```python
from build123d import *

# Parameters (mm, degrees)
SKETCH_1_W               = 15
SKETCH_1_H               = 15
EXTRUDE_1_DEPTH          = 5.5
CUT_EXTRUDE_1_DEPTH      = 11
EXTRUDE_2_DEPTH          = 2
EXTRUDE_2_DEPTH_BACK     = 2
CUT_EXTRUDE_2_DEPTH      = 2
CUT_EXTRUDE_2_DEPTH_BACK = 2
SKETCH_5_W               = 5.4
SKETCH_5_H               = 7.4
EXTRUDE_3_DEPTH          = 1
SKETCH_6_W               = 5.4
SKETCH_6_H               = 5
EXTRUDE_4_DEPTH          = 2
SKETCH_7_R               = 2
EXTRUDE_5_DEPTH          = 10
SKETCH_8_R               = 2.1
EXTRUDE_6_DEPTH          = 1
CHAMFER_1_SIZE           = 0.5
SKETCH_9_W               = 5
SKETCH_9_H               = 1
CUT_EXTRUDE_3_DEPTH      = 6
FILLET_1_R               = 0.1
FILLET_2_R               = 0.2


with BuildPart() as part:
    # 草图1 → 凸台-拉伸1 (new body)
    with BuildSketch(Plane(origin=(0, 0, 0), x_dir=(1, 0, 0), z_dir=(0, 1, 0))):
        Rectangle(SKETCH_1_W, SKETCH_1_H)
    extrude(amount=EXTRUDE_1_DEPTH)

    # 草图2 → 切除-拉伸1 (cut)
    with BuildSketch(Plane.XY.offset(7.5)):
        with BuildLine():
            Line((1.5, 0), (-1.5, 0))
            Line((-1.5, 0), (-1.5, 0.677124344))
            ThreePointArc((-1.5, 0.677124344), (0, 4), (1.5, 0.677124344))
            Line((1.5, 0.677124344), (1.5, 0))
        make_face()
    extrude(amount=-CUT_EXTRUDE_1_DEPTH, mode=Mode.SUBTRACT)

    # 草图3 → 凸台-拉伸2 (add, two sides: drawn at the far end of the back side and taken through both)
    with BuildSketch(Plane.XY.offset(-EXTRUDE_2_DEPTH_BACK)):
        with BuildLine():
            Line((1.5, 5.5), (-1.5, 5.5))
            Line((-1.5, 5.5), (-1.5, 6.177124344))
            ThreePointArc((-1.5, 6.177124344), (-1.780042303, 6.588161527), (-1.95, 7.055590279))
            Line((-1.95, 7.055590279), (-1.95, 8))
            Line((-1.95, 8), (1.95, 8))
            Line((1.95, 8), (1.95, 7.055590279))
            ThreePointArc((1.95, 7.055590279), (1.780042303, 6.588161527), (1.5, 6.177124344))
            Line((1.5, 6.177124344), (1.5, 5.5))
        make_face()
    extrude(amount=EXTRUDE_2_DEPTH + EXTRUDE_2_DEPTH_BACK)

    # 草图4 → 切除-拉伸2 (cut, two sides: drawn at the far end of the back side and taken through both)
    with BuildSketch(Plane(origin=(0, 0, 0), x_dir=(0, 0, -1), z_dir=(1, 0, 0)).offset(-CUT_EXTRUDE_2_DEPTH_BACK)):
        with BuildLine():
            Line((-1.5, 5.5), (-1.5, 6.177124344))
            ThreePointArc((-1.5, 6.177124344), (-1.780042303, 6.588161527), (-1.95, 7.055590279))
            Line((-1.95, 7.055590279), (-1.95, 8))
            Line((-1.95, 8), (-2, 8))
            Line((-2, 8), (-2, 5.5))
            Line((-2, 5.5), (-1.5, 5.5))
        make_face()
        with BuildLine():
            Line((2, 5.5), (1.5, 5.5))
            Line((1.5, 5.5), (1.5, 6.177124344))
            ThreePointArc((1.5, 6.177124344), (1.780042303, 6.588161527), (1.95, 7.055590279))
            Line((1.95, 7.055590279), (1.95, 8))
            Line((1.95, 8), (2, 8))
            Line((2, 8), (2, 5.5))
        make_face()
    extrude(amount=CUT_EXTRUDE_2_DEPTH + CUT_EXTRUDE_2_DEPTH_BACK, mode=Mode.SUBTRACT)

    # 草图5 → 凸台-拉伸3 (add)
    with BuildSketch(Plane(origin=(0, 0, -7.5), x_dir=(-1, 0, 0), z_dir=(0, 0, -1))):
        with Locations((0, 2.75)):
            Rectangle(SKETCH_5_W, SKETCH_5_H)
    extrude(amount=EXTRUDE_3_DEPTH)

    # 草图6 → 凸台-拉伸4 (add)
    with BuildSketch(Plane(origin=(0, 0, -8.5), x_dir=(-1, 0, 0), z_dir=(0, 0, -1))):
        with Locations((0, 2.5)):
            Rectangle(SKETCH_6_W, SKETCH_6_H)
    extrude(amount=EXTRUDE_4_DEPTH)

    # 草图7 → 凸台-拉伸5 (add)
    with BuildSketch(Plane(origin=(0, 0, -10.5), x_dir=(-1, 0, 0), z_dir=(0, 0, -1))):
        with Locations(Location((0, 2.2, 0), (0, 0, 180))):
            Circle(SKETCH_7_R)
    extrude(amount=EXTRUDE_5_DEPTH)

    # 草图8 → 凸台-拉伸6 (add)
    with BuildSketch(Plane(origin=(0, 0, -20.5), x_dir=(-1, 0, 0), z_dir=(0, 0, -1))):
        with Locations((0, 2.2)):
            Circle(SKETCH_8_R)
    extrude(amount=-EXTRUDE_6_DEPTH)

    # 倒角1
    chamfer_1_edges = [part.edges().sort_by_distance(p)[0] for p in [
        (2.1, 2.2, -20.5),
    ]]
    chamfer(chamfer_1_edges, length=CHAMFER_1_SIZE)

    # 草图9 → 切除-拉伸3 (cut)
    with BuildSketch(Plane(origin=(0, 0, -20.5), x_dir=(-1, 0, 0), z_dir=(0, 0, -1))):
        with Locations((0, 2.2)):
            Rectangle(SKETCH_9_W, SKETCH_9_H)
    extrude(amount=-CUT_EXTRUDE_3_DEPTH, mode=Mode.SUBTRACT)

    # 圆角1
    fillet_1_edges = [part.edges().sort_by_distance(p)[0] for p in [
        (1.95, 8, 0),
        (-1.95, 8, 0),
        (0, 8, -1.95),
        (0, 8, 1.95),
    ]]
    fillet(fillet_1_edges, radius=FILLET_1_R)

    # 圆角2
    fillet_2_edges = [part.edges().sort_by_distance(p)[0] for p in [
        (0, 5.5, 7.5),
        (-5.1, 0, -7.5),
        (-5.1, 5.5, -7.5),
        (-2.7, -0.95, -8),
        (0, 6.45, -7.5),
        (-2.7, 6.45, -8),
        (2.7, 6.45, -8),
        (0, -0.95, -7.5),
        (2.7, -0.95, -8),
        (-2.7, -0.475, -8.5),
        (0, 6.45, -8.5),
        (2.7, 5.725, -8.5),
        (0, -0.95, -8.5),
        (7.5, 5.5, 0),
        (-2.7, 5.725, -8.5),
        (2.7, -0.475, -8.5),
        (4.5, 0, 7.5),
        (2.7, 5, -9.5),
        (0, 0, -8.5),
        (2.7, 0, -9.5),
        (-2.7, 0, -9.5),
        (0, 5, -8.5),
        (-2.7, 5, -9.5),
        (2.7, 2.5, -10.5),
        (0, 0, -10.5),
        (-2.7, 2.5, -10.5),
        (0, 5, -10.5),
        (5.1, 5.5, -7.5),
        (7.5, 0, 0),
        (-4.5, 0, 7.5),
        (-7.5, 0, 0),
        (5.1, 0, -7.5),
        (-7.5, 5.5, 0),
        (7.5, 2.75, -7.5),
        (7.5, 2.75, 7.5),
        (-7.5, 2.75, 7.5),
        (-7.5, 2.75, -7.5),
    ]]
    fillet(fillet_2_edges, radius=FILLET_2_R - 0.0001)  # a hair under: the kernel refuses the full size


solid = part.part
```
Geometry: final body of the model. Coordinates: model frame, mm. A direction names the side the tool comes from. Coordinates: 2 decimals unless noted, no trailing zeros. Loops run counter-clockwise (first coordinate to the right, second up) from the corner with the lowest first, then second, coordinate; pieces in that order, holes last. Notation, with made-up numbers: (-8, 24.25) -> (49, 24.25) arc R17 ccw to (49, 52.25) -> close; hole circle Ø6 at (21.25, 19.25). An arc over 180 degrees is marked (long way). Use a Markdown table: item, result. Add a question column.
(1) Pin query (flat end, axial travel): pin 1 Ø0.6 at (x, y) = (0, 6) entering from +Z; pin 2 Ø1.5 at (x, z) = (-0.5, -3) entering from +Y; pin 3 Ø8 at (x, z) = (3.5, -17) entering from -Y. Return the tip coordinate at first contact, or that it passes through.
(2) Section query A-A, the plane z = -5.25. Return loops of the section in (x, y).
(3) Line query: line 1 along X through (y, z) = (2, 4.75); line 2 along Y through (x, z) = (0, 3.25); line 3 along Y through (x, z) = (0, 1). Output: solid intervals per line, ascending.
(4) Access query for faces 5 (the flat face through (-1.95, 7.5, 0)), 6 (the cylindrical face through (1.847, 2.966, -14.937)), 7 (the flat face through (1.95, 7.5, 0)), 8 (the flat face through (0, 5, -9)). Directions: +Z, -Z, +X, -X, +Y, -Y. A direction counts if a zero-diameter tool reaches every point of the face in a straight line with its end or side. Return the directions, or none.
(5) Section query C-C, the plane y = 2.2. Return loops of the section in (x, z), plus the area to 3 significant figures.
(6) Mould query, pull axis Y, two halves, no side actions, for faces 1 (the flat face through (0, 1, -20.5)), 2 (the cylindrical face through (-1.777, 6.582, -0.027)), 3 (the flat face through (0, 8, 0)), 4 (the flat face through (0, 2, -14.5)). Classes: pulls with the +Y half, pulls with the -Y half, needs draft (parallel to the pull), parting line crosses it, or undercut.
(7) Section query B-B, the plane x = 5. Return loops of the section in (y, z).
(8) Section query D-D, the plane z = -15.75. Return loops of the section in (x, y), plus the area to 3 significant figures.
Answer:
| question | item | result |
|---|---|---|
| 1 | pin 1 | stops at z = 1.6 |
| 1 | pin 2 | stops at y = 5.5 |
| 1 | pin 3 | stops at y = 0.13 |
| 2 | outline | (-7.5, 0.2) arc R0.2 ccw to (-7.3, 0) -> (7.3, 0) arc R0.2 ccw to (7.5, 0.2) -> (7.5, 5.3) arc R0.2 ccw to (7.3, 5.5) -> (-7.3, 5.5) arc R0.2 ccw to (-7.5, 5.3) -> close |
| 3 | line 1 | x = -7.5 to -2, 2 to 7.5 |
| 3 | line 2 | y = 4 to 5.5 |
| 3 | line 3 | y = 4 to 8 |
| 4 | face 5 | +Z, -Z, -X, +Y |
| 4 | face 6 | none |
| 4 | face 7 | +Z, -Z, +X, +Y |
| 4 | face 8 | -Z, +X, -X, +Y |
| 5 | outline | (-7.5, -7.3) arc R0.2 ccw to (-7.3, -7.5) -> (-2.7, -7.5) -> (-2.7, -10.3) arc R0.2 ccw to (-2.5, -10.5) -> (-2, -10.5) -> (-2, -14.5) -> (2, -14.5) -> (2, -10.5) -> (2.5, -10.5) arc R0.2 ccw to (2.7, -10.3) -> (2.7, -7.5) -> (7.3, -7.5) arc R0.2 ccw to (7.5, -7.3) -> (7.5, 7.3) arc R0.2 ccw to (7.3, 7.5) -> (1.99, 7.5) -> (1.99, -3.5) -> (-1.99, -3.5) -> (-1.99, 7.5) -> (-7.3, 7.5) arc R0.2 ccw to (-7.5, 7.3) -> close |
| 5 | area | 213 mm^2 |
| 6 | face 1 | needs draft |
| 6 | face 2 | undercut |
| 6 | face 3 | pulls with the +Y half |
| 6 | face 4 | undercut |
| 7 | outline | (0, -7.3) arc R0.2 ccw to (0.2, -7.5) -> (5.3, -7.5) arc R0.2 ccw to (5.5, -7.3) -> (5.5, 7.3) arc R0.2 ccw to (5.3, 7.5) -> (0.2, 7.5) arc R0.2 ccw to (0, 7.3) -> close |
| 8 | outline | (-1.94, 1.7) arc R2 ccw to (1.94, 1.7) -> close; (-1.94, 2.7) -> (1.94, 2.7) arc R2 ccw to start |
| 8 | area | 8.61 mm^2 |
